from build123d import *

# Parameters (mm, degrees)
F1_DEPTH = 40
F2_W     = 5.5
F2_H     = 5.5
F3_DEPTH = 11
F4_R     = 2
F5_R     = 1


# Not quite as in the source:
# - a feature names something its author has since deleted; it is built from what else it names


with BuildPart() as f1:
    # F0 (on Right) → F1 (new body, symmetric)
    with BuildSketch(Plane.YZ):
        with BuildLine():
            ThreePointArc((0, -18.25), (-12.9046987567, -12.9046987567), (-18.25, 0))
            Line((-18.25, 0), (-25, 0))
            Line((-25, 0), (-25, -80))
            Line((-25, -80), (21, -80))
            Line((21, -80), (21, -59))
            Line((21, -59), (11, -59))
            Line((11, -59), (11, -70))
            Line((11, -70), (0, -70))
            Line((0, -70), (0, -18.25))
        make_face()
        with BuildLine():
            Line((-13.25, 0), (-18.25, 0))
            ThreePointArc((-18.25, 0), (-12.9046987567, -12.9046987567), (0, -18.25))
            Line((0, -18.25), (0, -13.25))
            ThreePointArc((0, -13.25), (-9.3691648507, -9.3691648507), (-13.25, 0))
        make_face()
        with BuildLine():
            ThreePointArc((17.5517093185, -5), (18.0745842976, -2.5242627575), (18.25, 0))
            Line((18.25, 0), (13.25, 0))
            Line((13.25, 0), (13.25, -5))
            Line((13.25, -5), (17.5517093185, -5))
        make_face()
        with BuildLine():
            Line((18.25, -5), (18.25, 0))
            ThreePointArc((18.25, 0), (18.0745842976, -2.5242627575), (17.5517093185, -5))
            Line((17.5517093185, -5), (18.25, -5))
        make_face()
        with BuildLine():
            Line((13.25, 0), (18.25, 0))
            ThreePointArc((18.25, 0), (0, 18.25), (-18.25, 0))
            Line((-18.25, 0), (-13.25, 0))
            ThreePointArc((-13.25, 0), (0, 13.25), (13.25, 0))
        make_face()
    extrude(amount=F1_DEPTH, both=True)

    # F2 (on face) → F3 (cut)
    with BuildSketch(Plane(origin=(0, 0, 0), x_dir=(-1, 0, 0), z_dir=(0, 1, 0))):
        with Locations((-17.25, -29.25)):
            Rectangle(F2_W, F2_H)
        with Locations((-22.75, -29.25)):
            Rectangle(F2_W, F2_H)
        Polygon((-14.5, -32), (-20, -32), (-25.5, -32), (-25.5, -37.5), (-20, -37.5), (-14.5, -37.5), align=None)
        Polygon((25.5, -26.5), (20, -26.5), (14.5, -26.5), (14.5, -32), (14.5, -37.5), (20, -37.5), (25.5, -37.5), (25.5, -32), align=None)
    extrude(amount=-F3_DEPTH, mode=Mode.SUBTRACT)

    # F4
    f4_edges = [f1.edges().sort_by_distance(p)[0] for p in [
        (0, -18.25, 0),
    ]]
    fillet(f4_edges, radius=F4_R)

    # F5
    f5_edges = [f1.edges().sort_by_distance(p)[0] for p in [
        (-40, 0.902338, 18.227679),
        (-40, -18.808432, 0.517593),
        (-40, 18.25, -2.5),
        (-40, -22.575496, 0),
        (-40, 15.75, -5),
        (-40, -25, -40),
        (-40, 13.25, -2.5),
        (-40, -2, -80),
        (-40, -9.369165, 9.369165),
        (-40, 21, -69.5),
        (-40, 0, -41.625),
        (-40, 16, -59),
        (-40, 5.5, -70),
        (-40, 11, -64.5),
        (0, -25, -80),
        (40, -25, -40),
        (0, -25, 0),
        (40, 0.902338, 18.227679),
        (40, -18.808432, 0.517593),
        (40, 18.25, -2.5),
        (40, -22.575496, 0),
        (40, 15.75, -5),
        (40, 13.25, -2.5),
        (40, -2, -80),
        (40, -9.369165, 9.369165),
        (40, 21, -69.5),
        (40, 0, -41.625),
        (40, 16, -59),
        (40, 5.5, -70),
        (40, 11, -64.5),
        (0, 21, -80),
        (0, 21, -59),
        (0, 11, -59),
        (0, 18.25, -5),
        (0, 13.25, -5),
        (0, 0, -13.25),
        (25.5, 0, -32),
        (20, 0, -26.5),
        (14.5, 0, -32),
        (20, 0, -37.5),
        (-14.5, 0, -32),
        (-20, 0, -26.5),
        (-25.5, 0, -32),
        (-20, 0, -37.5),
    ]]
    fillet(f5_edges, radius=F5_R)


solid = f1.part
Read the model definition and answer for the solid it produces. Units are mm, in the model's axes. A direction names the side the tool comes from. Round coordinates to 2 decimals unless told otherwise and drop trailing zeros. Write each loop counter-clockwise with the first axis right and the second up, starting at its lowest first coordinate (ties: lowest second). Pieces come first, ordered by that corner, then holes. Notation, with made-up numbers: (13.5, -3) - (23.5, -3) arc R20 ccw to (23.5, 36) - close; hole circle Ø4 at (72, 13). An arc over 180 degrees is marked (long way). Use a Markdown table: item, result.
(1) Which of the six approach directions +Z, -Z, +X, -X, +Y, -Y give full straight-line access (tool end or side, diameter ignored) to faces 4 (the flat face through (1, 16, -59)), 5 (the flat face through (-20, -11, -32)), 6 (the flat face through (1, 18.25, -2))?
Reported:
| item | result |
|---|---|
| face 4 | +X, -X, +Y |
| face 5 | +Y |
| face 6 | +Z, +X, -X, +Y |
(2) The mould has two halves that part along Z. Classify faces 1 (the flat face through (-25.5, -6, -32)), 2 (the flat face through (1, 21, -70)), 3 (the cylindrical face through (0.546, 1.29, 18.204)): released by +Z, released by -Z, zero draft, split by the parting line, or undercut.
Reported:
| item | result |
|---|---|
| face 1 | undercut |
| face 2 | zero draft |
| face 3 | released by +Z |
(3) Each of these flat-tipped pins is pushed along its axis until it touches: pin 1 Ø3.5 at (x, z) = (-22, -31) entering from +Y; pin 2 Ø3 at (x, y) = (20.5, -7.5) entering from +Z; pin 3 Ø3 at (x, y) = (-2.5, 6.5) entering from +Z. Where does it stop, or does it pass through?
Reported:
| item | result |
|---|---|
| pin 1 | y = -11 |
| pin 2 | z = 17.24 |
| pin 3 | z = 17.55 |
(4) Straight lines are drawn through the part: line 1 along X through (y, z) = (-5, -29); line 2 along Z through (x, y) = (12, -22.5); line 3 along Y through (x, z) = (-4.5, -51). For each, find the intervals that lie inside material, in ascending order. Write a range as [from, to].
Reported:
| item | result |
|---|---|
| line 1 | [-40, -25.5], [-14.5, 14.5], [25.5, 40] |
| line 2 | [-80, 0] |
| line 3 | [-25, 0] |
(5) The part is cut by section A-A (z = -67). Write down the section's boundary in (x, y).
Reported:
| item | result |
|---|---|
| outline | (-40, -24) arc R1 ccw to (-39, -25) - (39, -25) arc R1 ccw to (40, -24) - (40, -1) arc R1 ccw to (39, 0) - (-39, 0) arc R1 ccw to (-40, -1) - close; (-40, 12) arc R1 ccw to (-39, 11) - (39, 11) arc R1 ccw to (40, 12) - (40, 20) arc R1 ccw to (39, 21) - (-39, 21) arc R1 ccw to (-40, 20) - close |
(6) The part is cut by section B-B (x = 17). Write down the section's boundary in (y, z).
Reported:
| item | result |
|---|---|
| outline | (-25, -79) arc R1 ccw to (-24, -80) - (20, -80) arc R1 ccw to (21, -79) - (21, -60) arc R1 ccw to (20, -59) - (12, -59) arc R1 ccw to (11, -60) - (11, -70) - (0, -70) - (0, -38.5) arc R1 ccw to (-1, -37.5) - (-11, -37.5) - (-11, -26.5) - (-1, -26.5) arc R1 ccw to (0, -25.5) - (0, -14.21) arc R1 ccw to (-0.93, -13.22) arc R13.25 cw (long way) to (13.25, 0) - (13.25, -4) arc R1 ccw to (14.25, -5) - (17.25, -5) arc R1 ccw to (18.25, -4) - (18.25, 0) arc R18.25 ccw to (-18.16, 1.8) arc R2 cw to (-20.15, 0) - (-24, 0) arc R1 ccw to (-25, -1) - close |
